Answer from the drawing. Dimensions are ordinates in mm from the lowest x, y and z of the part. Round coordinates to 2 decimals unless told otherwise and drop trailing zeros. Order: outer loops, then holes, each group sorted by start corner. A loop starts at its lowest first (then second) coordinate and runs counter-clockwise, first axis right, second up. Notation, with made-up numbers: M 77,74 L 115,74 A15 ccw 115,100 Z; hole C 25,40.25 d6. An arc over 180 degrees is marked long. Write item = value, one per line. Start each with the question number.
(1) For a pull along X with two mould halves and no side action, classify the marked faces 1 and 2 as released by +X, released by -X, zero draft, split by the parting line, or undercut.
(2) A cutting plane is placed at B-B, the plane x = 12. Determine the outline of the cut face in (y, z), and give its area (3 significant figures).
(3) Straight lines are drawn through the part: probe 1 along Y at (x, z) = (59, 2.55); probe 2 along Y at (x, z) = (58, 3) (1 decimal). For each, find the intervals that lie inside material, in ascending order. Write a range as from..to.
(4) A cutting plane is placed at C-C, the plane y = 54. Determine the outline of the cut face in (x, z).
(5) Each of these flat-tipped pins is pushed along its axis until it touches: pin 1 (2 mm diameter, centred on x = 8, z = 4.5, fed in from +Y); pin 2 (1.5 mm diameter, centred on x = 44, z = 5, fed in from -Y); pin 3 (1 mm diameter, centred on y = 14, z = 1.5, fed in from +X). Where does it stop, or does it pass through?
(6) A cutting plane is placed at A-A, the plane z = 3.7. Determine the outline of the cut face in (x, y).
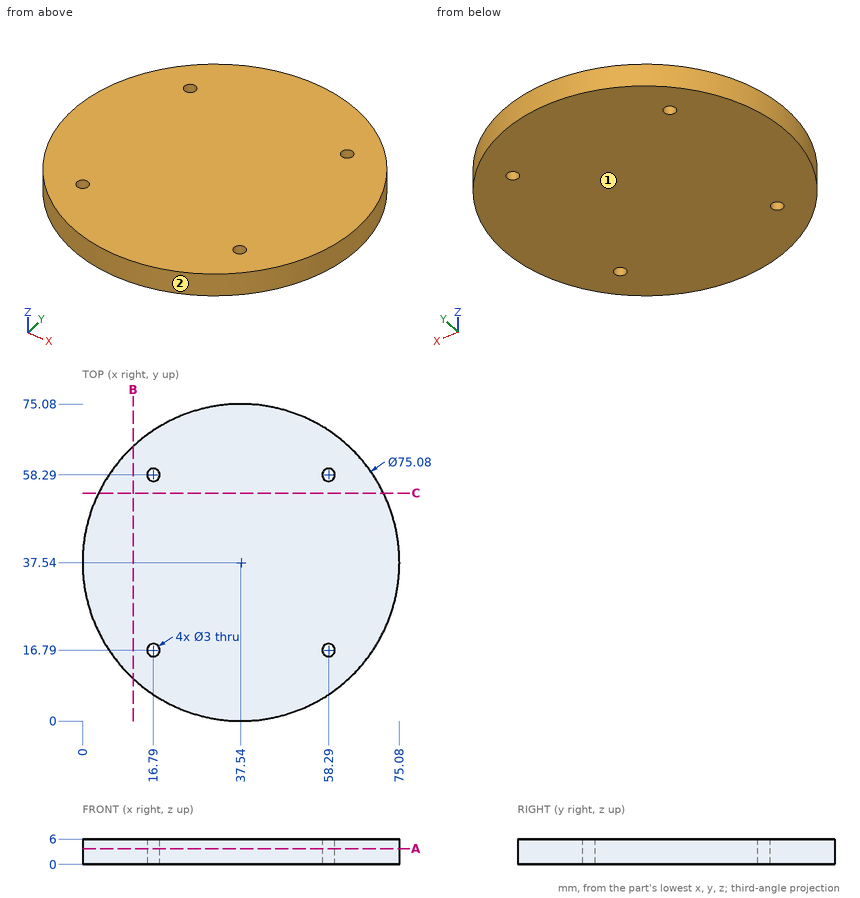
Reported:
q1.face_1 = zero draft
q1.face_2 = split by the parting line
q2.outline = M 10.03,0 L 65.05,0 L 65.05,6 L 10.03,6 Z
q2.area = 330 mm²
q3.probe_1 = 6.74..15.47, 18.11..56.97, 59.61..68.34
q3.probe_2 = 6.1..15.3, 18.3..56.8, 59.8..69
q4.outline = M 3.8,0 L 71.28,0 L 71.28,6 L 3.8,6 Z
q5.pin_1 = 61.93
q5.pin_2 = 0.44
q5.pin_3 = 67.18
q6.outline = C 37.54,37.54 d75.08; hole C 16.79,16.79 d3; hole C 16.79,58.29 d3; hole C 58.29,16.79 d3; hole C 58.29,58.29 d3
